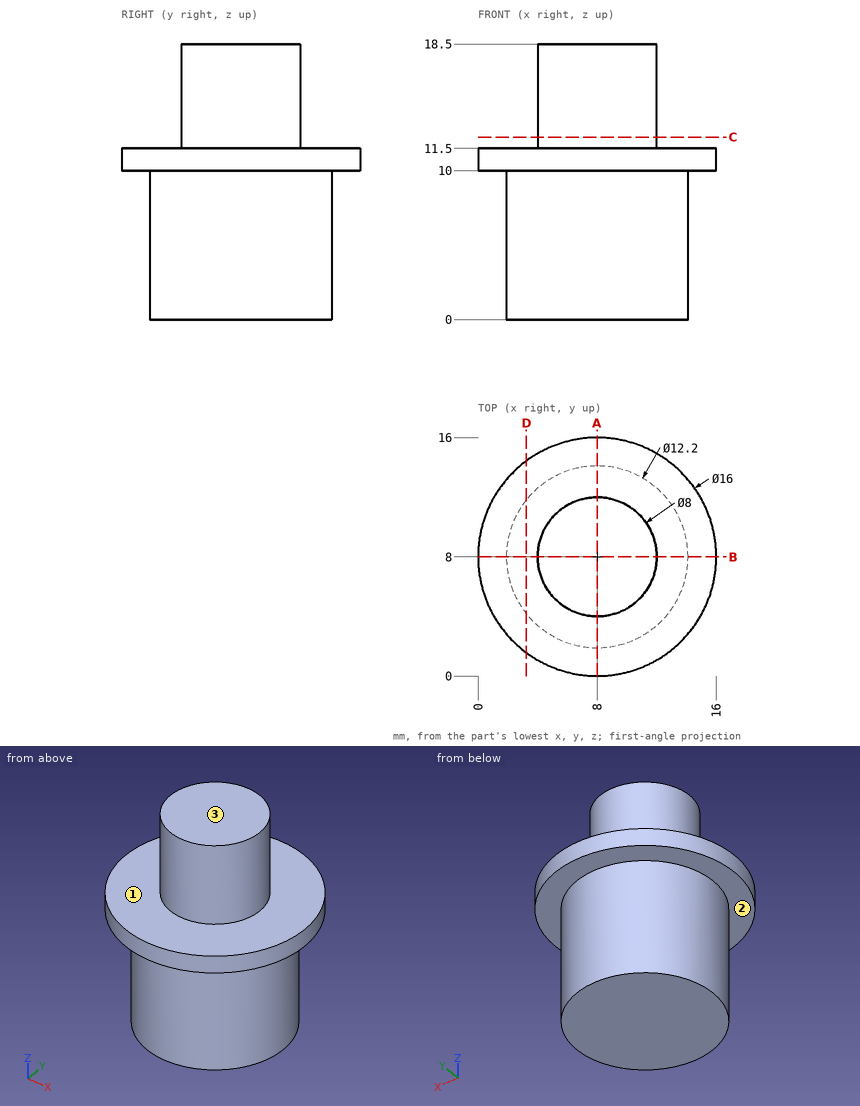
Answer from the drawing. Dimensions are ordinates in mm from the lowest x, y and z of the part. A direction names the side the tool comes from. Give positions to 0.01 mm unless a question says otherwise; leave off trailing zeros. Order: outer loops, then holes, each group sorted by start corner. A loop starts at its lowest first (then second) coordinate and runs counter-clockwise, first axis right, second up.
Item 1: Find the intervals of material crossed by probe 1 along Z at (x, y) = (12, 3); probe 2 along Z at (x, y) = (4.75, 12.25); probe 3 along X at (y, z) = (8.75, 14.25), in increasing order.
From the geometry:
probe 1: z = 10 to 11.5
probe 2: z = 0 to 11.5
probe 3: x = 4.07 to 11.93
Item 2: The part is cut by section A-A, the plane x = 8. Give the vertices of the cut face in (y, z).
From the geometry:
outline: (0, 10) - (1.9, 10) - (1.9, 0) - (14.1, 0) - (14.1, 10) - (16, 10) - (16, 11.5) - (12, 11.5) - (12, 18.5) - (4, 18.5) - (4, 11.5) - (0, 11.5) - close
Item 3: Given pin 1 Ø2 at (x, z) = (11.5, 4) entering from +Y; pin 2 Ø1 at (x, z) = (11, 3) entering from -Y; pin 3 Ø5 at (x, z) = (5, 2.5) entering from -Y, each flat-ended and moving along its own axis, determine where each tip first touches the part or whether it passes through.
From the geometry:
pin 1: stops at y = 13.56
pin 2: stops at y = 2.44
pin 3: stops at y = 1.92
Item 4: The part is cut by section C-C, the plane z = 12.25. Give the vertices of the cut face in (x, y).
From the geometry:
outline: circle Ø8 at (8, 8)
Item 5: Which of the six approach directions +Z, -Z, +X, -X, +Y, -Y give full straight-line access (tool end or side, diameter ignored) to the marked faces 1, 2 and 3?
From the geometry:
face 1: +Z
face 2: -Z
face 3: +Z, +X, -X, +Y, -Y
Item 6: The part is cut by section D-D, the plane x = 3.25. Give the vertices of the cut face in (y, z), and give its area (3 significant figures).
From the geometry:
outline: (1.56, 10) - (4.17, 10) - (4.17, 0) - (11.83, 0) - (11.83, 10) - (14.44, 10) - (14.44, 11.5) - (1.56, 11.5) - close
area: 95.9 mm2
